The listing builds one solid part. Answer for the finished solid, in the listing's coordinates (mm). Give positions to 0.01 mm unless a question says otherwise; leave off trailing zeros. Order: outer loops, then holes, each group sorted by start corner. A loop starts at its lowest first (then second) coordinate and runs counter-clockwise, first axis right, second up. Notation, with made-up numbers: (83, 61.25) - (125, 61.25) arc R37 cw to (125, 100.25) - close; hole circle Ø8 at (35, -22). An arc over 180 degrees is marked (long way). Answer as CSV lines item,"result". Start each with the question number.
1. Section B-B on x = 50.8 is taken. Count the separate pieces of the cut face and the enclosed holes in it, and give its area (3 significant figures).
2. Section C-C on x = -68.5 is taken. Give the vertices of the cut face in (y, z), and give its area (3 significant figures).
3. Consider line 1 along Z through (x, y) = (-127, -0.5); line 2 along Z through (x, y) = (50.8, -0.75) (3 decimals); line 3 along Z through (x, y) = (-17.5, -0.85) (3 decimals). Determine where each line is inside the solid, lowest interval first. Write a range as [from, to].
4. Section A-A on z = 31.75 is taken. Give the vertices of the cut face in (x, y) (1 decimal).
5. Flat-ended cylindrical pins translate along their axes: pin 1 (4 mm diameter, centred on x = -35.72, z = -30.52, fed in from -Y); pin 2 (1.5 mm diameter, centred on x = -31.5, z = -48, fed in from +Y). Find the tip coordinate at first contact, or state that the pin passes through.
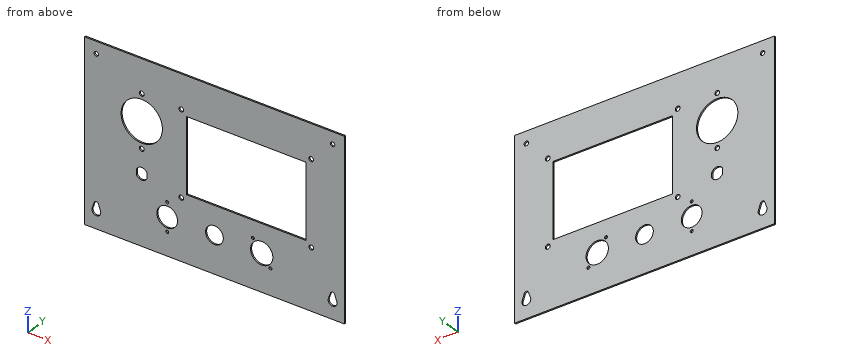
from build123d import *

# Parameters (mm, degrees)
F0_W     = 279.4
F0_H     = 190.5
F1_DEPTH = 1.5875
F2_W     = 128.5875
F2_H     = 79.375
F2_R     = 2.54
F3_DEPTH = 25.4
F4_R     = 22.225
F4_R_2   = 2.54
F5_DEPTH = 25.4
F6_R     = 12.0015
F6_R_2   = 1.5875
F6_R_3   = 9.525
F6_R_4   = 11.1125
F7_DEPTH = 25.4
F8_R     = 2.38125
F9_DEPTH = 25.4


with BuildPart() as f1:
    # F0 (on Front) → F1 (new body)
    with BuildSketch(Plane.XZ):
        Rectangle(F0_W, F0_H)
    extrude(amount=F1_DEPTH)

    # F2 (on face) → F3 (cut)
    with BuildSketch(Plane.XZ.offset(1.5875)):
        with Locations((34.13125, 14.2875)):
            Rectangle(F2_W, F2_H)
        with Locations((-35.71875, 59.09945)):
            Circle(F2_R)
        with Locations((103.98125, 59.09945)):
            Circle(F2_R)
        with Locations((103.98125, -30.52445)):
            Circle(F2_R)
        with Locations((-35.71875, -30.52445)):
            Circle(F2_R)
    extrude(amount=-F3_DEPTH, mode=Mode.SUBTRACT)

    # F4 (on face) → F5 (cut)
    with BuildSketch(Plane.XZ.offset(1.5875)):
        with Locations((-78.184375, 31.75)):
            Circle(F4_R)
        with Locations((-78.184375, 59.69)):
            Circle(F4_R_2)
        with Locations((-78.184375, 3.81)):
            Circle(F4_R_2)
    extrude(amount=-F5_DEPTH, mode=Mode.SUBTRACT)

    # F6 (on face) → F7 (cut)
    with BuildSketch(Plane.XZ.offset(1.5875)):
        with Locations((50.8, -55.5625)):
            Circle(F6_R)
        with Locations((41.3385, -43.561)):
            Circle(F6_R_2)
        with Locations((60.2615, -67.564)):
            Circle(F6_R_2)
        with Locations((0, -55.5625)):
            Circle(F6_R_3)
        with BuildLine():
            Line((-84.039075, -18.940748), (-84.039075, -24.239252))
            ThreePointArc((-84.039075, -24.239252), (-78.184375, -28.0162), (-72.329675, -24.239252))
            Line((-72.329675, -24.239252), (-72.329675, -18.940748))
            ThreePointArc((-72.329675, -18.940748), (-78.184375, -15.1638), (-84.039075, -18.940748))
        make_face()
        with Locations((-50.8, -55.5625)):
            Circle(F6_R_4)
        with Locations((-50.8, -40.48125)):
            Circle(F6_R_2)
        with Locations((-50.8, -70.64375)):
            Circle(F6_R_2)
    extrude(amount=-F7_DEPTH, mode=Mode.SUBTRACT)

    # F8 (on face) → F9 (cut)
    with BuildSketch(Plane.XZ.offset(1.5875)):
        with Locations((-127, 82.55)):
            Circle(F8_R)
        with Locations((127, 82.55)):
            Circle(F8_R)
        with BuildLine():
            Line((-122.509872, -75.40625), (-124.754936, -69.05625))
            ThreePointArc((-124.754936, -69.05625), (-127, -67.46875), (-129.245064, -69.05625))
            Line((-129.245064, -69.05625), (-131.490128, -75.40625))
            ThreePointArc((-131.490128, -75.40625), (-127, -81.75625), (-122.509872, -75.40625))
        make_face()
        with BuildLine():
            Line((131.490128, -75.40625), (129.245064, -69.05625))
            ThreePointArc((129.245064, -69.05625), (127, -67.46875), (124.754936, -69.05625))
            Line((124.754936, -69.05625), (122.509872, -75.40625))
            ThreePointArc((122.509872, -75.40625), (127, -81.75625), (131.490128, -75.40625))
        make_face()
    extrude(amount=-F9_DEPTH, mode=Mode.SUBTRACT)


solid = f1.part
Checks:
1,separate pieces,"3"
1,enclosed holes,"0"
1,area,"138 mm²"
2,outline,"(-1.59, -95.25) - (0, -95.25) - (0, 11.75) - (-1.59, 11.75) - close; (-1.59, 51.75) - (0, 51.75) - (0, 95.25) - (-1.59, 95.25) - close"
2,area,"239 mm²"
3,line 1,"z = [-95.25, -81.76], [-67.47, 80.17], [84.93, 95.25]"
3,line 2,"z = [-95.25, -67.564], [-43.561, -25.4], [53.975, 95.25]"
3,line 3,"z = [-95.25, -25.4], [53.975, 95.25]"
4,outline,"(-139.7, -1.6) - (-100.4, -1.6) - (-100.4, 0) - (-139.7, 0) - close; (-56, -1.6) - (-30.2, -1.6) - (-30.2, 0) - (-56, 0) - close; (98.4, -1.6) - (139.7, -1.6) - (139.7, 0) - (98.4, 0) - close"
5,pin 1,"passes through"
5,pin 2,"stops at y = 0"
